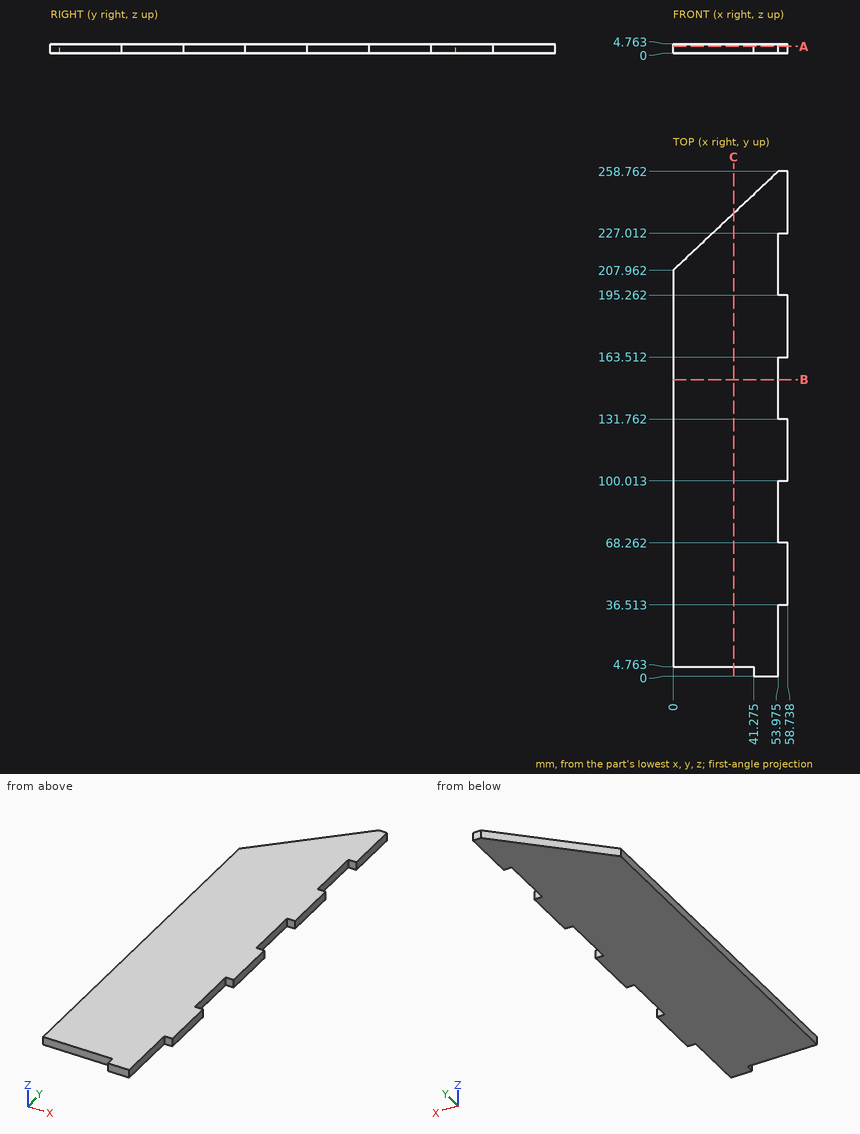
The drawing under review shows one solid part. Ordinate dimensions are in mm from its lowest x, y, z. Round coordinates to 2 decimals unless told otherwise and drop trailing zeros. Loops run counter-clockwise (first coordinate to the right, second up) from the corner with the lowest first, then second, coordinate; pieces in that order, holes last. Notation, with made-up numbers: (-30.5, 73) - (-18.5, 73) arc R20 ccw to (-18.5, 109) - close; hole circle Ø7 at (45.25, 68). An arc over 180 degrees is marked (long way). One line per question, with ' | ' between items.
Q1. Take a section at B-B (y = 152). Give the boundary of the cut face in (x, z) (1 decimal), and give its area (3 significant figures).
Taken from the geometry:
outline: (0, 0) - (54, 0) - (54, 4.8) - (0, 4.8) - close | area: 257 mm²
Q2. Take a section at A-A (z = 3.6). Give the boundary of the cut face in (x, y) (1 decimal).
Taken from the geometry:
outline: (0, 4.8) - (41.3, 4.8) - (41.3, 0) - (54, 0) - (54, 36.5) - (58.7, 36.5) - (58.7, 68.3) - (54, 68.3) - (54, 100) - (58.7, 100) - (58.7, 131.8) - (54, 131.8) - (54, 163.5) - (58.7, 163.5) - (58.7, 195.3) - (54, 195.3) - (54, 227) - (58.7, 227) - (58.7, 258.8) - (54, 258.8) - (0, 208) - close
Q3. For pin 1 (2.5 mm diameter, centred on x = 28, z = 1.5, fed in from -Y); pin 2 (1.4 mm diameter, centred on y = 3.5, z = 2, fed in from -X) (1 decimal); pin 3 (2.5 mm diameter, centred on x = 56, z = 1.5, fed in from -Y), all flat-tipped, find the tip position at first contact; note any pin that passes through.
Taken from the geometry:
pin 1: stops at y = 4.76 | pin 2: stops at x = 41.3 | pin 3: stops at y = 36.51
Q4. For line 1 along X through (y, z) = (77, 0.4) (1 decimal); line 2 along Y through (x, z) = (51, 2.1) (1 decimal); line 3 along Y through (x, z) = (39, 1.15) (1 decimal), list the stretches that pass through material, from the lowest coordinate up. Write a range as [from, to].
Taken from the geometry:
line 1: x = [0, 54] | line 2: y = [0, 256] | line 3: y = [4.8, 244.7]
Q5. Take a section at C-C (x = 31). Give the boundary of the cut face in (y, z), and give its area (3 significant figures).
Taken from the geometry:
outline: (4.76, 0) - (237.14, 0) - (237.14, 4.76) - (4.76, 4.76) - close | area: 1,110 mm²
